```python
from build123d import *

# Parameters (mm, degrees)
SKETCH1_R           = 7.5
BOSS_EXTRUDE1_DEPTH = 6
SKETCH2_R           = 7.5
SKETCH2_R_2         = 6.366385485
CUT_EXTRUDE1_DEPTH  = 5
SKETCH3_R           = 2.5
CUT_EXTRUDE2_DEPTH  = 6


with BuildPart() as part:
    # Sketch1 → Boss-Extrude1 (new, symmetric)
    with BuildSketch(Plane.XY):
        Circle(SKETCH1_R)
    extrude(amount=BOSS_EXTRUDE1_DEPTH, both=True)

    # Sketch2 → Cut-Extrude1 (cut, symmetric)
    with BuildSketch(Plane.XY):
        Circle(SKETCH2_R)
        Circle(SKETCH2_R_2, mode=Mode.SUBTRACT)
    extrude(amount=CUT_EXTRUDE1_DEPTH, both=True, mode=Mode.SUBTRACT)

    # Sketch3 → Cut-Extrude2 (cut, symmetric)
    with BuildSketch(Plane.XY):
        Circle(SKETCH3_R)
    extrude(amount=CUT_EXTRUDE2_DEPTH, both=True, mode=Mode.SUBTRACT)


solid = part.part
```
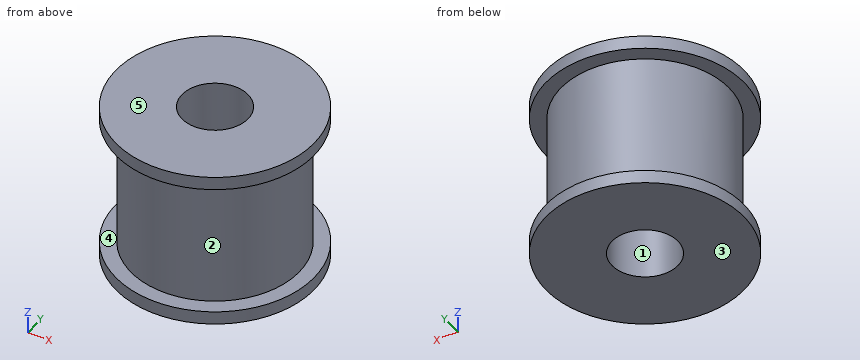
Geometry: final body of the model. Coordinates: model frame, mm. Face numbers are marked on the shaded views. A direction names the side the tool comes from. Coordinates: 2 decimals unless noted, no trailing zeros. Loops run counter-clockwise (first coordinate to the right, second up) from the corner with the lowest first, then second, coordinate; pieces in that order, holes last. Notation, with made-up numbers: (29.5, 30) -> (58.5, 30) arc R9 cw to (58.5, 42) -> close; hole circle Ø7 at (-25.75, 5.25). An arc over 180 degrees is marked (long way). Use a Markdown table: item, result. Add a question column.
(1) Pin query (flat end, axial travel): pin 1 Ø2 at (x, z) = (2.5, -3) entering from -Y; pin 2 Ø4 at (y, z) = (-2.5, 0.5) entering from +X; pin 3 Ø3 at (y, z) = (-5, 2.5) entering from -X. Return the tip coordinate at first contact, or that it passes through.
(2) Section query D-D, the plane y = 4.75. Return loops of the section in (x, z).
(3) Access query for the marked faces 4 and 5. Directions: +Z, -Z, +X, -X, +Y, -Y. A direction counts if a zero-diameter tool reaches every point of the face in a straight line with its end or side. Return the directions, or none.
(4) Section query C-C, the plane z = 4.25. Return loops of the section in (x, y), plus the area to 3 significant figures.
(5) Section query A-A, the plane y = 0. Return loops of the section in (x, z), plus the area to 3 significant figures.
(6) Line query: line 1 along Y through (x, z) = (0, 3); line 2 along X through (y, z) = (-4.25, -3.75); line 3 along X through (y, z) = (-1.5, -5.25). Output: solid intervals per line, ascending.
(7) Mould query, pull axis X, two halves, no side actions, for the marked faces 1, 2 and 3. Classes: pulls with the +X half, pulls with the -X half, needs draft (parallel to the pull), parting line crosses it, or undercut.
Answer:
| question | item | result |
|---|---|---|
| 1 | pin 1 | stops at y = -6.19 |
| 1 | pin 2 | stops at x = 6.35 |
| 1 | pin 3 | stops at x = -5.32 |
| 2 | outline | (-5.8, -6) -> (5.8, -6) -> (5.8, -5) -> (4.24, -5) -> (4.24, 5) -> (5.8, 5) -> (5.8, 6) -> (-5.8, 6) -> (-5.8, 5) -> (-4.24, 5) -> (-4.24, -5) -> (-5.8, -5) -> close |
| 3 | face 4 | none |
| 3 | face 5 | +Z, +X, -X, +Y, -Y |
| 4 | outline | circle Ø12.73 at (0, 0); hole circle Ø5 at (0, 0) |
| 4 | area | 108 mm^2 |
| 5 | outline | (-7.5, -6) -> (-2.5, -6) -> (-2.5, 6) -> (-7.5, 6) -> (-7.5, 5) -> (-6.37, 5) -> (-6.37, -5) -> (-7.5, -5) -> close; (2.5, -6) -> (7.5, -6) -> (7.5, -5) -> (6.37, -5) -> (6.37, 5) -> (7.5, 5) -> (7.5, 6) -> (2.5, 6) -> close |
| 5 | area | 97.3 mm^2 |
| 6 | line 1 | y = -6.37 to -2.5, 2.5 to 6.37 |
| 6 | line 2 | x = -4.74 to 4.74 |
| 6 | line 3 | x = -7.35 to -2, 2 to 7.35 |
| 7 | face 1 | undercut |
| 7 | face 2 | parting line crosses it |
| 7 | face 3 | needs draft |
